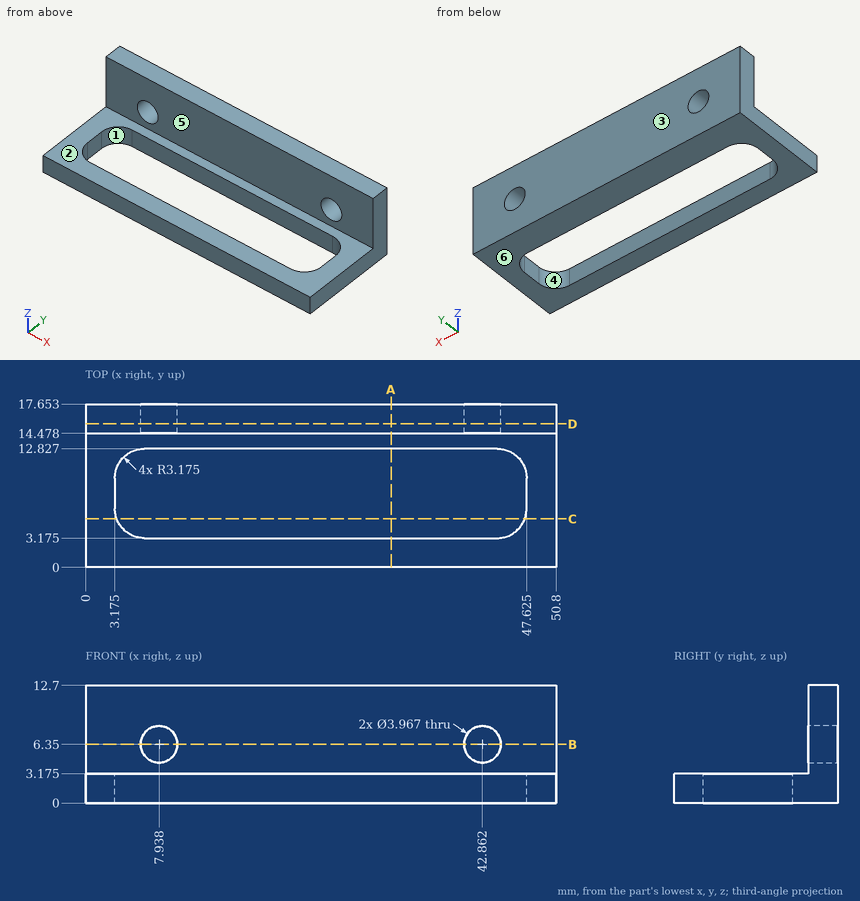
For this review, use the dimensioned drawing (mm, ordinates from the lowest corner) and the shaded views. A direction names the side the tool comes from. Give positions to 0.01 mm unless a question says otherwise; leave off trailing zeros. Write each loop counter-clockwise with the first axis right and the second up, starting at its lowest first coordinate (ties: lowest second). Pieces come first, ordered by that corner, then holes. Notation, with made-up numbers: M 70,54 L 91,54 A13 cw 91,69 Z; hole C -22,28.5 d9. An arc over 180 degrees is marked long. Answer as a JSON object with one key per item and string values. Group by question number.
Item 1: Consider section C-C on y = 5.25. Write out the cut boundary in (x, z) (1 decimal).
Item 2: Consider section B-B on z = 6.35. Write out the cut boundary in (x, y).
Item 3: Consider section A-A on x = 33. Write out the cut boundary in (y, z) (1 decimal).
Item 4: Consider section D-D on y = 15.5. Write out the cut boundary in (x, z).
Item 5: Draft analysis for pull direction Y (two halves, no side actions). For the marked faces 1, 2, 3 and 4, state which applies: +Y half, -Y half, draft (parallel to the pull), parting line (faces both ways), or undercut.
Item 6: For pin 1 Ø3 at (x, z) = (31.5, 8.5) entering from -Y; pin 2 Ø3.5 at (y, z) = (8.5, 2) entering from -X, all flat-tipped, find the tip position at first contact; note any pin that passes through.
Item 7: For probe 1 along X at (y, z) = (15.35, 6.35); probe 2 along Y at (x, z) = (33, 3) (1 decimal); probe 3 along Y at (x, z) = (9, 3.75), list the stretches that pass through material, from the lowest coordinate up. Write a range as [from, to].
Item 8: Tool access review of the marked faces 5 and 6: name each direction out of +Z, -Z, +X, -X, +Y, -Y from which nothing blocks a thin tool from reaching the whole face with its end or side.
Check result:
{
 "1": {"outline": "M 0,0 L 3.4,0 L 3.4,3.2 L 0,3.2 Z; M 47.4,0 L 50.8,0 L 50.8,3.2 L 47.4,3.2 Z"},
 "2": {"outline": "M 0,14.48 L 5.95,14.48 L 5.95,17.65 L 0,17.65 Z; M 9.92,14.48 L 40.88,14.48 L 40.88,17.65 L 9.92,17.65 Z; M 44.85,14.48 L 50.8,14.48 L 50.8,17.65 L 44.85,17.65 Z"},
 "3": {"outline": "M 0,0 L 3.2,0 L 3.2,3.2 L 0,3.2 Z; M 12.8,0 L 17.7,0 L 17.7,12.7 L 14.5,12.7 L 14.5,3.2 L 12.8,3.2 Z"},
 "4": {"outline": "M 0,0 L 50.8,0 L 50.8,12.7 L 0,12.7 Z; hole C 7.94,6.35 d3.97; hole C 42.86,6.35 d3.97"},
 "5": {"face 1": "undercut", "face 2": "draft", "face 3": "+Y half", "face 4": "undercut"},
 "6": {"pin 1": "stops at y = 14.48", "pin 2": "stops at x = 0"},
 "7": {"probe 1": "x = [0, 5.95], [9.92, 40.88], [44.85, 50.8]", "probe 2": "y = [0, 3.2], [12.8, 17.7]", "probe 3": "y = [14.48, 17.65]"},
 "8": {"face 5": "+Z, +X, -X, -Y", "face 6": "-Z, +X, -X, +Y, -Y"}
}
